For this review, take the finished solid that the model builds, in its own axes (mm). Face numbers are marked on the shaded views. A direction names the side the tool comes from. Give positions to 0.01 mm unless a question says otherwise; leave off trailing zeros. Loops run counter-clockwise (first coordinate to the right, second up) from the corner with the lowest first, then second, coordinate; pieces in that order, holes last.
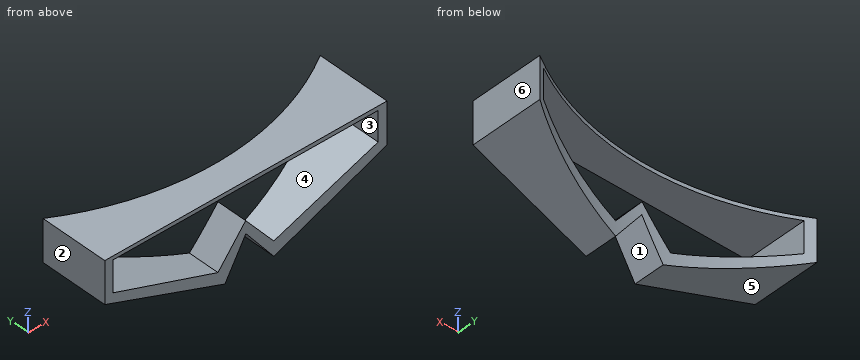
```python
from build123d import *

# Parameters (mm, degrees)
F1_DEPTH = 146
F3_DEPTH = 60
F5_DEPTH = 500


with BuildPart() as f1:
    # F0 (on Front) → F1 (new body)
    with BuildSketch(Plane.XZ):
        Polygon((-3.734913, 26.905388), (-3.734913, 51.905388), (-88.734913, 51.905388), (-173.734913, 51.905388), (-173.734913, 26.905388), (-101.347528, 0), (-88.734913, 21.905388), (-71.878783, 0), align=None)
    extrude(amount=F1_DEPTH)

    # F2 (on face) → F3 (cut)
    with BuildSketch(Plane.XY.offset(51.905388)):
        with BuildLine():
            Line((-173.734913, 0), (-173.734913, -105.142423))
            ThreePointArc((-173.734913, -105.142423), (-88.257826, -127.680535), (-3.734913, -101.792774))
            Line((-3.734913, -101.792774), (-3.734913, 0))
            Line((-3.734913, 0), (-173.734913, 0))
        make_face()
    extrude(amount=-F3_DEPTH, mode=Mode.SUBTRACT)

    # F4 (on face) → F5 (cut)
    with BuildSketch(Plane.XZ.offset(146)):
        Polygon((-9.079793, 49.414322), (-168.665886, 49.675085), (-168.665886, 30.900249), (-105.561584, 8.735513), (-88.872842, 29.335679), (-71.923338, 8.735513), (-9.079793, 31.421773), align=None)
    extrude(amount=-F5_DEPTH, mode=Mode.SUBTRACT)


solid = f1.part
```
Item 1: Take a section at C-C on x = -29.5. Give the boundary of the cut face in (y, z).
Answer:
outline: (-146, 16.73) - (-115.35, 16.73) - (-115.35, 24.05) - (-146, 24.05) - close; (-146, 49.45) - (-115.35, 49.45) - (-115.35, 51.91) - (-146, 51.91) - close
Item 2: For L1, parallel to X at y = -118.5, z = 34; L2, parallel to Z at x = -163, y = -134; L3, parallel to Z at x = -29.5, y = -123.5, list the stretches that pass through material, from the lowest coordinate up.
Answer:
L1: x = -173.73 to -168.67, -9.08 to -3.73
L2: z = 22.92 to 28.91, 49.67 to 51.91
L3: z = 16.73 to 24.05, 49.45 to 51.91
Item 3: Take a section at A-A on z = 41.5. Give the boundary of the cut face in (x, y), and give its area (3 significant figures).
Answer:
outline: (-173.73, -146) - (-168.67, -146) - (-168.67, -108.03) arc R161.33 cw to (-173.73, -105.14) - close; (-9.08, -146) - (-3.73, -146) - (-3.73, -101.79) arc R161.33 cw to (-9.08, -105.11) - close
area: 427 mm2
Item 4: Take a section at B-B on y = -115.5. Give the boundary of the cut face in (x, z).
Answer:
outline: (-173.73, 26.91) - (-153.01, 19.2) - (-153.01, 25.4) - (-168.67, 30.9) - (-168.67, 49.68) - (-153.01, 49.65) - (-153.01, 51.91) - (-173.73, 51.91) - close; (-29.86, 16.59) - (-3.73, 26.91) - (-3.73, 51.91) - (-29.86, 51.91) - (-29.86, 49.45) - (-9.08, 49.41) - (-9.08, 31.42) - (-29.86, 23.92) - close
Item 5: Clearance check with flat-ended pins moving along their axes: pin 1 Ø3 at (x, z) = (-26.5, 20.5) entering from +Y; pin 2 Ø2 at (x, y) = (-148, -134.5) entering from -Z. State where each tip first meets the part, or that it passes through.
Answer:
pin 1: stops at y = -113.4
pin 2: stops at z = 16.97
Item 6: Tool access review of the marked faces 1, 2 and 3: name each direction out of +Z, -Z, +X, -X, +Y, -Y from which nothing blocks a thin tool from reaching the whole face with its end or side.
Answer:
face 1: -Z, +Y, -Y
face 2: +Z, -Z, -X, +Y, -Y
face 3: +Y, -Y
Item 7: Take a section at D-D on y = -130.5. Give the boundary of the cut face in (x, z).
Answer:
outline: (-173.73, 26.91) - (-101.35, 0) - (-88.73, 21.91) - (-71.88, 0) - (-3.73, 26.91) - (-3.73, 51.91) - (-173.73, 51.91) - close; hole (-168.67, 30.9) - (-105.56, 8.74) - (-88.87, 29.34) - (-71.92, 8.74) - (-9.08, 31.42) - (-9.08, 49.41) - (-168.67, 49.68) - close
Item 8: The part is to be moulded in two halves that separate along Z. For the marked faces 4, 5 and 6, say which applies: released by +Z, released by -Z, zero draft, split by the parting line, or undercut.
Answer:
face 4: undercut
face 5: released by -Z
face 6: zero draft
